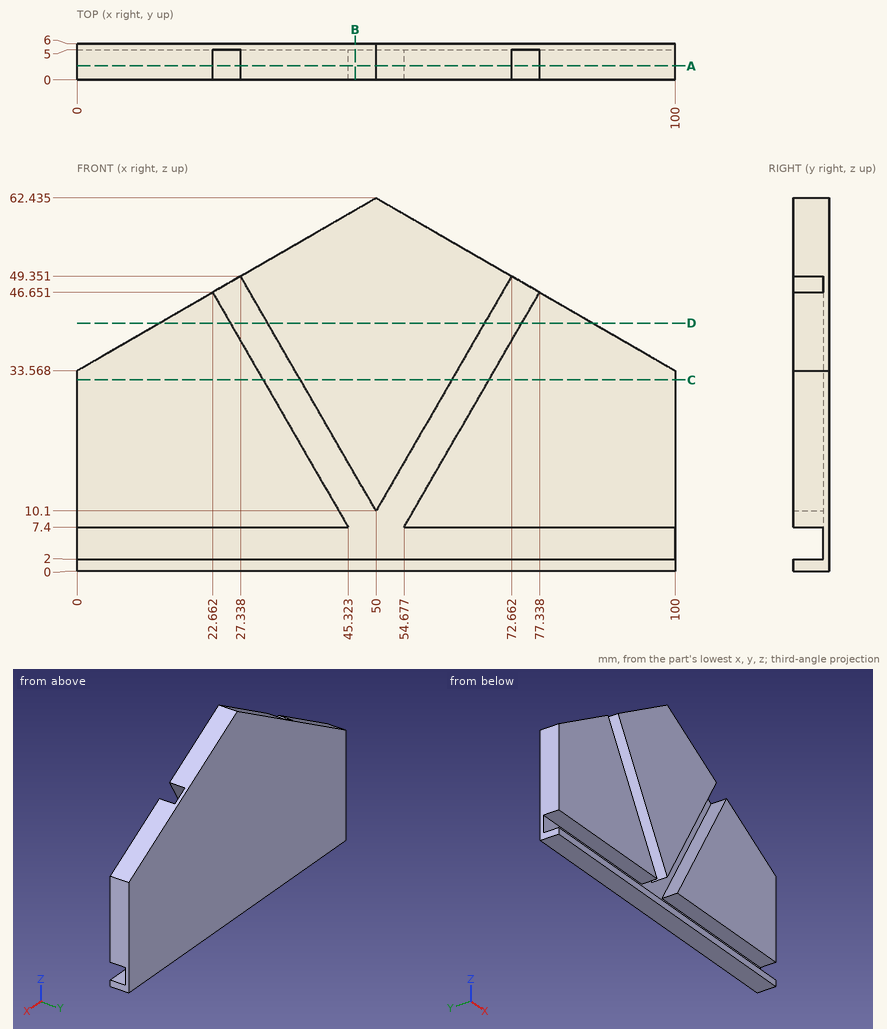
Geometry: see drawing. Coordinates: mm, zero at the bounding-box minimum. Round coordinates to 2 decimals unless told otherwise and drop trailing zeros. Loops run counter-clockwise (first coordinate to the right, second up) from the corner with the lowest first, then second, coordinate; pieces in that order, holes last. Notation, with made-up numbers: M 82,23 L 114,23 A27 cw 114,43 Z; hole C -9.75,35 d2. An arc over 180 degrees is marked long. Use a Markdown table: item, result. Add a question column.
1. Section query B-B on x = 46.5. Return the cut outline in (y, z) (1 decimal), then the cut area to 3 significant figures.
2. Contact query for a flat-ended pin moving along its axis: P1, Ø1.5, axis at y = 3.5, z = 14.5, coming from the -X side. Output: stop coordinate, or through.
3. Line query: line 1 (X direction, y = 2.65, z = 26.5) (1 decimal); line 2 (X direction, y = 1.6, z = 19.5) (1 decimal); line 3 (Z direction, x = 44, y = 2.6) (1 decimal). Output: solid intervals per line, ascending.
4. Section query D-D on z = 41.5. Return the cut outline in (x, y) (1 decimal), then the cut area to 3 significant figures.
5. Section query C-C on z = 32. Return the cut outline in (x, y).
6. Section query A-A on y = 2.35. Return the cut outline in (x, z) (1 decimal).
Reported:
| question | item | result |
|---|---|---|
| 1 | outline | M 0,0 L 6,0 L 6,60.4 L 0,60.4 L 0,16.2 L 5,16.2 L 5,2 L 0,2 Z |
| 1 | area | 292 mm² |
| 2 | P1 | stops at x = 0 |
| 3 | line 1 | x = 0 to 34.3, 40.5 to 59.5, 65.7 to 100 |
| 3 | line 2 | x = 0 to 38.3, 44.6 to 55.4, 61.7 to 100 |
| 3 | line 3 | z = 0 to 2, 7.4 to 9.7, 20.5 to 59 |
| 4 | outline | M 13.7,0 L 25.6,0 L 25.6,5 L 31.9,5 L 31.9,0 L 68.1,0 L 68.1,5 L 74.4,5 L 74.4,0 L 86.3,0 L 86.3,6 L 13.7,6 Z |
| 4 | area | 373 mm² |
| 5 | outline | M 0,0 L 31.12,0 L 31.12,5 L 37.36,5 L 37.36,0 L 62.64,0 L 62.64,5 L 68.88,5 L 68.88,0 L 100,0 L 100,6 L 0,6 Z |
| 6 | outline | M 0,0 L 100,0 L 100,2 L 0,2 Z; M 0,7.4 L 45.3,7.4 L 22.7,46.7 L 0,33.6 Z; M 27.3,49.4 L 50,10.1 L 72.7,49.4 L 50,62.4 Z; M 54.7,7.4 L 100,7.4 L 100,33.6 L 77.3,46.7 Z |
